```python
from build123d import *

# Parameters (mm, degrees)
SKETCH1_W               = 35
SKETCH1_H               = 35
BOSS_EXTRUDE1_DEPTH     = 3
SKETCH3_R               = 1.8
CUT_EXTRUDE2_DEPTH      = 3
MIRROR2_COPY_1_SKETCH_R = 1.8
MIRROR2_COPY_1_DEPTH    = 3
SKETCH2_R               = 2.7
BOSS_EXTRUDE2_DEPTH     = 5
BOSS_EXTRUDE3_DEPTH     = 3
FILLET2_R               = 0.5
FILLET3_R               = 2
FILLET4_R               = 5


with BuildPart() as part:
    # Sketch1 → Boss-Extrude1 (new body)
    with BuildSketch(Plane(origin=(0, 0, 0), x_dir=(1, 0, 0), z_dir=(0, 1, 0))):
        with Locations((17.5, 17.5)):
            Rectangle(SKETCH1_W, SKETCH1_H)
    extrude(amount=BOSS_EXTRUDE1_DEPTH)

    # Sketch3 → Cut-Extrude2 (cut)
    with BuildSketch(Plane(origin=(0, 3, 0), x_dir=(1, 0, 0), z_dir=(0, 1, 0))):
        with Locations(Location((3, 21, 0), (0, 0, 270))):
            Circle(SKETCH3_R)
    cut_extrude2 = extrude(amount=-CUT_EXTRUDE2_DEPTH, mode=Mode.SUBTRACT)

    # Mirror1: Cut-Extrude2 across plane
    add(cut_extrude2.mirror(Plane.XY.offset(-12.5)), mode=Mode.SUBTRACT)

    # Mirror2: Cut-Extrude2 across plane
    add(cut_extrude2.mirror(Plane(origin=(17.5, 0, 0), x_dir=(0, 0, 1), z_dir=(1, 0, 0))), mode=Mode.SUBTRACT)

    # Mirror2 copy 1 sketch → Mirror2 copy 1 (cut)
    with BuildSketch(Plane(origin=(35, 3, -25), x_dir=(-1, 0, 0), z_dir=(0, 1, 0))):
        with Locations(Location((3, 21, 0), (0, 0, 270))):
            Circle(MIRROR2_COPY_1_SKETCH_R)
    extrude(amount=-MIRROR2_COPY_1_DEPTH, mode=Mode.SUBTRACT)

    # Sketch2 → Boss-Extrude2 (add)
    with BuildSketch(Plane(origin=(0, 3, 0), x_dir=(1, 0, 0), z_dir=(0, 1, 0))):
        with Locations(Location((17.5, 15, 0), (0, 0, 90))):
            Circle(SKETCH2_R)
    extrude(amount=BOSS_EXTRUDE2_DEPTH)

    # Sketch5 → Boss-Extrude3 (add)
    with BuildSketch(Plane(origin=(0, 3, 0), x_dir=(1, 0, 0), z_dir=(0, 1, 0))):
        Polygon((17.5, 4.5), (15.5, 0), (19.5, 0), align=None)
    extrude(amount=BOSS_EXTRUDE3_DEPTH)

    # Fillet2
    fillet2_edges = [part.edges().sort_by_distance(p)[0] for p in [
        (17.5, 4.5, -4.5),
    ]]
    fillet(fillet2_edges, radius=FILLET2_R)

    # Fillet3
    fillet3_edges = [part.edges().sort_by_distance(p)[0] for p in [
        (35, 1.5, 0),
        (0, 1.5, 0),
    ]]
    fillet(fillet3_edges, radius=FILLET3_R)

    # Fillet4
    fillet4_edges = [part.edges().sort_by_distance(p)[0] for p in [
        (0, 1.5, -35),
        (35, 1.5, -35),
    ]]
    fillet(fillet4_edges, radius=FILLET4_R)


solid = part.part
```
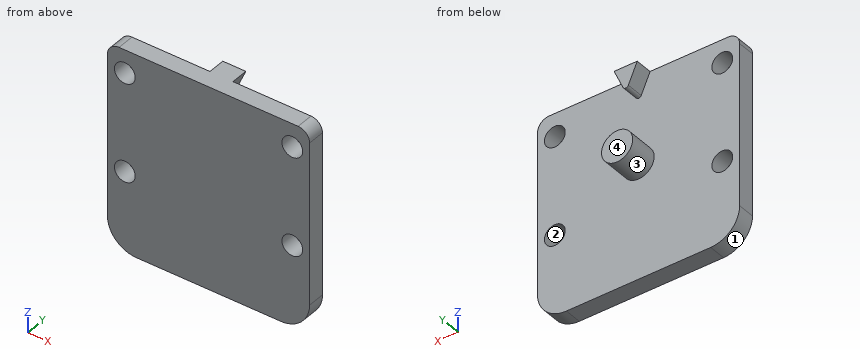
Check sheet for the modelled part. Datum: model origin and axes. Units: mm. Face numbers are marked on the shaded views. Round coordinates to 2 decimals unless told otherwise and drop trailing zeros. Order: outer loops, then holes, each group sorted by start corner. A loop starts at its lowest first (then second) coordinate and runs counter-clockwise, first axis right, second up.
1) Mould release check, pull along X, two halves, no side actions. Record for the marked faces 1, 2, 3 and 4: +X half, -X half, draft (parallel to the pull), parting line (faces both ways), or undercut.
2) Section check B-B (z = -21). Record the boundary of the cut face in (x, y), and give its area (3 significant figures).
3) Section check D-D (x = 17.5). Record the boundary of the cut face in (y, z).
4) Go/stop test with flat-tipped pins: pin 1 Ø4 at (x, z) = (3, -21) entering from -Y; pin 2 Ø1.1 at (x, z) = (17.5, -2.5) entering from +Y; pin 3 Ø1.5 at (x, z) = (19, -20) entering from +Y. Record where each tip stops, or that it passes through.
5) Section check A-A (y = 5.5). Record the boundary of the cut face in (x, z).
6) Scan lines: line 1 (X direction, y = 1, z = -21); line 2 (Z direction, x = 32, y = 1.6); line 3 (Y direction, x = 13.5, z = -6). Record each from-to range of solid material in increasing order.
7) Section check C-C (x = 32). Record the boundary of the cut face in (y, z).
Result:
1. face 1: -X half
1. face 2: undercut
1. face 3: parting line
1. face 4: draft
2. outline: (0, 0) - (1.2, 0) - (1.2, 3) - (0, 3) - close; (4.8, 0) - (30.2, 0) - (30.2, 3) - (4.8, 3) - close; (33.8, 0) - (35, 0) - (35, 3) - (33.8, 3) - close
2. area: 83.4 mm2
3. outline: (0, -35) - (3, -35) - (3, -17.7) - (8, -17.7) - (8, -12.3) - (3, -12.3) - (3, -3.77) - (6, -3.77) - (6, 0) - (0, 0) - close
4. pin 1: stops at y = 0
4. pin 2: stops at y = 6
4. pin 3: stops at y = 3
5. outline: circle Ø5.4 at (17.5, -15); (15.5, 0) - (17.04, -3.47) arc R0.5 ccw to (17.96, -3.47) - (19.5, 0) - close
6. line 1: x = 0 to 1.2, 4.8 to 30.2, 33.8 to 35
6. line 2: z = -34.58 to -22.8, -19.2 to -5.8, -2.2 to 0
6. line 3: y = 0 to 3
7. outline: (0, -34.58) - (3, -34.58) - (3, -22.8) - (0, -22.8) - close; (0, -19.2) - (3, -19.2) - (3, -5.8) - (0, -5.8) - close; (0, -2.2) - (3, -2.2) - (3, 0) - (0, 0) - close
